CAD build for the part. Positions are in the model's coordinates, mm. Coordinates: 2 decimals unless noted, no trailing zeros. Loops run counter-clockwise (first coordinate to the right, second up) from the corner with the lowest first, then second, coordinate; pieces in that order, holes last. Notation, with made-up numbers: (81.25, 52) -> (123.25, 52) arc R15 ccw to (123.25, 67) -> close; hole circle Ø11 at (46, 77.25). An arc over 180 degrees is marked (long way). Return JSON: item names as keys, results as strings. Group by question number.
(1) Saw through at A-A on x = 20.5. Write the cut outline in (y, z).
(2) Probe L1, parallel to Y at x = 5, z = 0.5; L2, parallel to X at y = -8, z = 0.35; L3, parallel to X at y = 12, z = 0.2. List the from-to ranges inside material, lowest first.
(3) Saw through at B-B on y = 11. Write the cut outline in (x, z).
(4) Flat gauge pins, fed straight in: pin 1 Ø6 at (x, y) = (17.5, 2.5) entering from +Z; pin 2 Ø0.5 at (y, z) = (19, 0.5) entering from -X. Where does each tip first touch, or does it go through?
(5) Mould opens along Y. For faces 1 (the face through (15, 7, 0)), 2 (the face through (37.12, -2.14, 0.49)) say: pulls with the +Y half, pulls with the -Y half, needs draft (parallel to the pull), parting line crosses it, or undercut.
(6) Saw through at C-C on y = -3.5. Write the cut outline in (x, z), then the cut area to 3 significant figures.
(7) Saw through at D-D on z = 0.8. Write the cut outline in (x, y) (3 decimals), then the cut area to 3 significant figures.
```python
from build123d import *

# Parameters (mm, degrees)
CROQUIS1_R              = 1.25
CROQUIS1_R_2            = 2.625
CROQUIS1_R_3            = 1.5
CROQUIS1_W              = 22.5
CROQUIS1_H              = 11.8
CROQUIS1_W_2            = 12
CROQUIS1_H_2            = 7
SALIENTE_EXTRUIR1_DEPTH = 1


with BuildPart() as part:
    # Croquis1 → Saliente-Extruir1 (new body)
    with BuildSketch(Plane.XY):
        Polygon((0.682906484, 8.504854369), (0.682906484, 35.504854369), (16.682906484, 35.504854369), (16.682906484, 8.504854369), (40.690737834, 8.504854369), (40.690737834, -11.495145631), (-10.607093516, -11.495145631), (-10.607093516, 8.504854369), align=None)
        with Locations((8.682906484, 31.504854369)):
            Circle(CROQUIS1_R, mode=Mode.SUBTRACT)
        with Locations((-5.323911872, -2.595145631)):
            Circle(CROQUIS1_R_2, mode=Mode.SUBTRACT)
        with Locations((35.690737834, -2.595145631)):
            Circle(CROQUIS1_R_3, mode=Mode.SUBTRACT)
        with Locations((15.926088128, -2.595145631)):
            Rectangle(CROQUIS1_W, CROQUIS1_H, mode=Mode.SUBTRACT)
        with Locations((8.682906484, 9.246132474)):
            Rectangle(CROQUIS1_W_2, CROQUIS1_H_2, mode=Mode.SUBTRACT)
    extrude(amount=SALIENTE_EXTRUIR1_DEPTH)


solid = part.part
```
Geometry results:
{
 "1": {"outline": "(-11.5, 0) -> (-8.5, 0) -> (-8.5, 1) -> (-11.5, 1) -> close; (3.3, 0) -> (8.5, 0) -> (8.5, 1) -> (3.3, 1) -> close"},
 "2": {"L1": "-11.5 to -8.5, 3.3 to 5.75, 12.75 to 35.5", "L2": "-10.61 to 4.68, 27.18 to 40.69", "L3": "0.68 to 2.68, 14.68 to 16.68"},
 "3": {"outline": "(0.68, 0) -> (2.68, 0) -> (2.68, 1) -> (0.68, 1) -> close; (14.68, 0) -> (16.68, 0) -> (16.68, 1) -> (14.68, 1) -> close"},
 "4": {"pin 1": "z = 1", "pin 2": "x = 0.68"},
 "5": {"face 1": "needs draft", "face 2": "undercut"},
 "6": {"outline": "(-10.61, 0) -> (-7.79, 0) -> (-7.79, 1) -> (-10.61, 1) -> close; (-2.86, 0) -> (4.68, 0) -> (4.68, 1) -> (-2.86, 1) -> close; (27.18, 0) -> (34.49, 0) -> (34.49, 1) -> (27.18, 1) -> close; (36.89, 0) -> (40.69, 0) -> (40.69, 1) -> (36.89, 1) -> close", "area": "21.5 mm²"},
 "7": {"outline": "(-10.607, -11.495) -> (40.691, -11.495) -> (40.691, 8.505) -> (16.683, 8.505) -> (16.683, 35.505) -> (0.683, 35.505) -> (0.683, 8.505) -> (-10.607, 8.505) -> close; hole circle Ø5.25 at (-5.324, -2.595); hole (2.683, 5.746) -> (14.683, 5.746) -> (14.683, 12.746) -> (2.683, 12.746) -> close; hole (4.676, -8.495) -> (27.176, -8.495) -> (27.176, 3.305) -> (4.676, 3.305) -> close; hole circle Ø2.5 at (8.683, 31.505); hole circle Ø3 at (35.691, -2.595)", "area": "1,070 mm²"}
}
